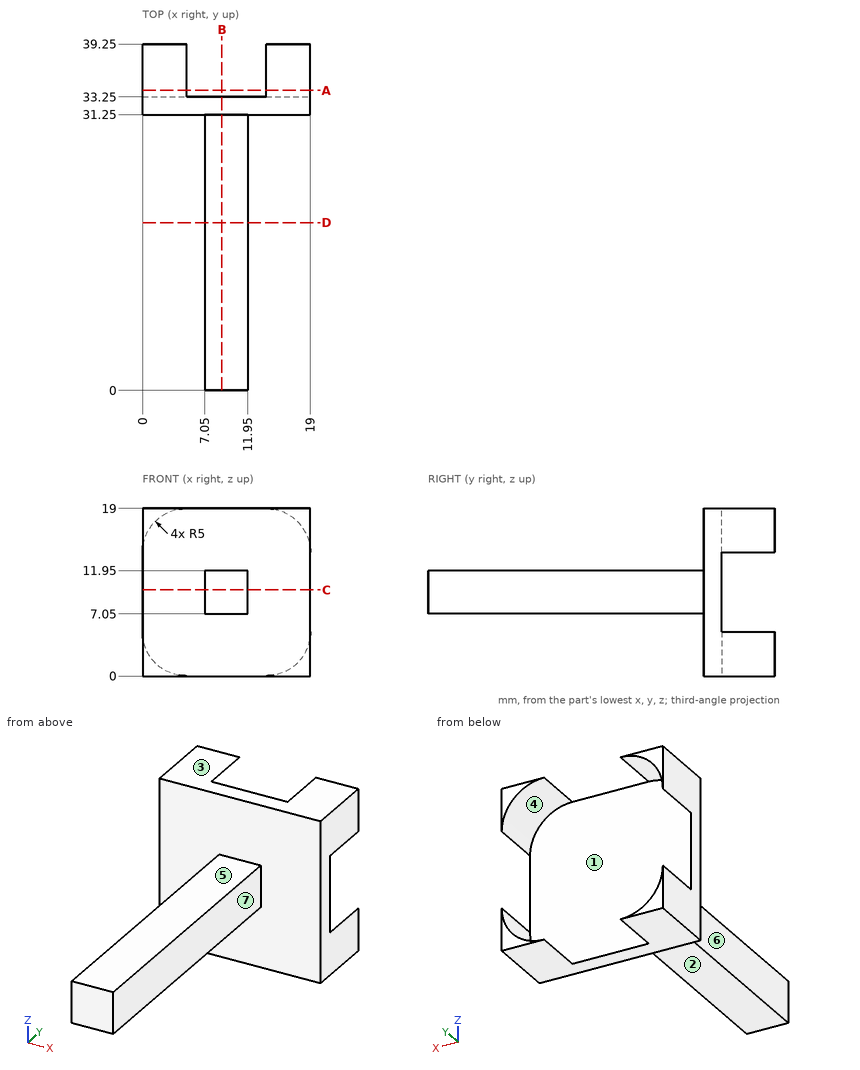
Can you work these out from the drawing? Everything is in mm from the part's minimum corner. A direction names the side the tool comes from. Give positions to 0.01 mm unless a question says otherwise; leave off trailing zeros. Loops run counter-clockwise (first coordinate to the right, second up) from the corner with the lowest first, then second, coordinate; pieces in that order, holes last. Notation, with made-up numbers: M 46.5,56.25 L 58.5,56.25 A23 cw 58.5,68.25 Z; hole C -36,3 d5. An arc over 180 degrees is marked long. Use CSV: the item, a comma, the result in double quotes. Start each with the question number.
1. Imagine slicing it at B-B, the plane x = 9. Write out the boundary of the cut face in (y, z), plus the area to 3 significant figures.
2. For P1, Ø2.5, axis at y = 20.5, z = 10, coming from the +X side; P2, Ø1.5, axis at y = 15.5, z = 8.5, coming from the -X side; P3, Ø4, axis at x = 5.5, y = 29, coming from the +Z side; P4, Ø1, axis at y = 6.5, z = 14, coming from the -X side, each with a flat end and sliding along its axis, tell me the tip position at first contact or that it passes through.
3. Imagine slicing it at A-A, the plane y = 34. Write out the boundary of the cut face in (x, z), plus the area to 3 significant figures.
4. If I drill on L1, parallel to X at y = 31, z = 11; L2, parallel to Y at x = 6.5, z = 17.5, over which ranges is the centre line in solid material (lowest first)?
5. Imagine slicing it at D-D, the plane y = 19. Write out the boundary of the cut face in (x, z).
6. Imagine slicing it at C-C, the plane z = 9.75. Write out the boundary of the cut face in (x, y).
7. If we mould it in two halves opening along Z, with no side actions, what happens to the marked faces 1, 2 and 3? For each: released by +Z, released by -Z, zero draft, split by the parting line, or undercut.
8. On a 3-axis mill with a long thin cutter (end or side, diameter ignored), from which of +Z, -Z, +X, -X, +Y, -Y can I reach the whole of each face in a straight line? I mean the marked faces 4, 5, 6 and 7. Say none if no direction works.
Response values:
1,outline,"M 0,7.05 L 31.25,7.05 L 31.25,0 L 33.25,0 L 33.25,19 L 31.25,19 L 31.25,11.95 L 0,11.95 Z"
1,area,"191 mm^2"
2,P1,"x = 11.95"
2,P2,"x = 7.05"
2,P3,"z = 11.95"
2,P4,"through"
3,outline,"M 0,0 L 5,0 A5 cw 0,5 Z; M 0,14 A5 cw 5,19 L 0,19 Z; M 14,0 L 19,0 L 19,5 A5 cw Z; M 14,19 A5 cw 19,14 L 19,19 Z"
3,area,"21.5 mm^2"
4,L1,"7.05 to 11.95"
4,L2,"31.25 to 33.25"
5,outline,"M 7.05,7.05 L 11.95,7.05 L 11.95,11.95 L 7.05,11.95 Z"
6,outline,"M 0,31.25 L 7.05,31.25 L 7.05,0 L 11.95,0 L 11.95,31.25 L 19,31.25 L 19,33.25 L 0,33.25 Z"
7,face 1,"undercut"
7,face 2,"released by -Z"
7,face 3,"released by +Z"
8,face 4,"+Y"
8,face 5,"+Z, +X, -X, -Y"
8,face 6,"+Z, -Z, -X, -Y"
8,face 7,"+Z, -Z, +X, -Y"
